from build123d import *

# Parameters (mm, degrees)
SKETCH_2_R          = 5
EXTRUDE_1_DEPTH     = 16
SKETCH_3_R          = 8
EXTRUDE_2_DEPTH     = 7
SKETCH_4_R          = 4
EXTRUDE_3_DEPTH     = 13.25
CUT_EXTRUDE_1_DEPTH = 3
CHAMFER_1_SIZE      = 0.5
SKETCH_6_R          = 4
SKETCH_6_R_2        = 3.5
CUT_EXTRUDE_2_DEPTH = 1


with BuildPart() as part:
    # 草图2 → 凸台-拉伸1 (new body)
    with BuildSketch(Plane.XY):
        Circle(SKETCH_2_R)
    extrude(amount=EXTRUDE_1_DEPTH)

    # 草图3 → 凸台-拉伸2 (add)
    with BuildSketch(Plane.XY.offset(16)):
        Circle(SKETCH_3_R)
    extrude(amount=EXTRUDE_2_DEPTH)

    # 草图4 → 凸台-拉伸3 (add)
    with BuildSketch(Plane(origin=(0, 0, 0), x_dir=(-1, 0, 0), z_dir=(0, 0, -1))):
        Circle(SKETCH_4_R)
    extrude(amount=EXTRUDE_3_DEPTH)

    # 草图5 → 切除-拉伸1 (cut)
    with BuildSketch(Plane.XY.offset(23)):
        Polygon((0, 5.456235198), (-4.72523829, 2.728117599), (-4.72523829, -2.728117599), (0, -5.456235198), (4.72523829, -2.728117599), (4.72523829, 2.728117599), align=None)
    extrude(amount=-CUT_EXTRUDE_1_DEPTH, mode=Mode.SUBTRACT)

    # 倒角1
    chamfer_1_edges = [part.edges().sort_by_distance(p)[0] for p in [
        (4, 0, -13.25),
    ]]
    chamfer(chamfer_1_edges, length=CHAMFER_1_SIZE)

    # 草图6 → 切除-拉伸2 (cut)
    with BuildSketch(Plane(origin=(0, 0, 0), x_dir=(-1, 0, 0), z_dir=(0, 0, -1))):
        Circle(SKETCH_6_R)
        Circle(SKETCH_6_R_2, mode=Mode.SUBTRACT)
    extrude(amount=CUT_EXTRUDE_2_DEPTH, mode=Mode.SUBTRACT)


solid = part.part
Geometry check sheet. Reference: the model listing, model coordinates, mm. A direction names the side the tool comes from. Give positions to 0.01 mm unless a question says otherwise; leave off trailing zeros. Write each loop counter-clockwise with the first axis right and the second up, starting at its lowest first coordinate (ties: lowest second). Pieces come first, ordered by that corner, then holes. Notation, with made-up numbers: (-5.5, 34.25) - (52.5, 34.25) arc R24 ccw to (52.5, 65.25) - close; hole circle Ø1 at (1.5, -21.5). An arc over 180 degrees is marked (long way). Put each result on its own line as item: value.
1. Sectioned sample at D-D, the plane y = 4.5. Enter the section's corners in (x, z).
Ans:
outline: (-6.61, 16) - (-2.18, 16) - (-2.18, 0) - (2.18, 0) - (2.18, 16) - (6.61, 16) - (6.61, 23) - (1.66, 23) - (1.66, 20) - (-1.66, 20) - (-1.66, 23) - (-6.61, 23) - close
2. Sectioned sample at B-B, the plane z = 18. Enter the section's corners in (x, y), plus the area to 3 significant figures.
Ans:
outline: circle Ø16 at (0, 0)
area: 201 mm²
3. Thickness scan on line 1 (Z direction, x = -1.5, y = -4); line 2 (Z direction, x = -2.75, y = 5); line 3 (Y direction, x = -3, z = 21). Record the ranges inside material, lowest first.
Ans:
line 1: z = 0 to 20
line 2: z = 16 to 23
line 3: y = -7.42 to -3.72, 3.72 to 7.42
4. Sectioned sample at A-A, the plane y = 0. Enter the section's corners in (x, z).
Ans:
outline: (-8, 16) - (-5, 16) - (-5, 0) - (-3.5, 0) - (-3.5, -1) - (-4, -1) - (-4, -12.75) - (-3.5, -13.25) - (3.5, -13.25) - (4, -12.75) - (4, -1) - (3.5, -1) - (3.5, 0) - (5, 0) - (5, 16) - (8, 16) - (8, 23) - (4.73, 23) - (4.73, 20) - (-4.73, 20) - (-4.73, 23) - (-8, 23) - close
5. Go/stop test with flat-tipped pins: pin 1 (5 mm diameter, centred on y = -1.5, z = -5, fed in from -X); pin 2 (6 mm diameter, centred on x = 1.5, z = 3, fed in from +Y); pin 3 (7.5 mm diameter, centred on x = 1.5, y = -2.5, fed in from +Z); pin 4 (5 mm diameter, centred on x = -3, z = 17, fed in from +Y). Record where each tip stops, or that it passes through.
Ans:
pin 1: stops at x = -4
pin 2: stops at y = 5
pin 3: stops at z = 23
pin 4: stops at y = 7.98
6. Sectioned sample at C-C, the plane x = 6. Enter the section's corners in (y, z).
Ans:
outline: (-5.29, 16) - (5.29, 16) - (5.29, 23) - (-5.29, 23) - close
7. Draft check along X on faces 5 (the flat face through (0, 0, 20)), 6 (the cylindrical face through (-1.73, -7.81, 19.45)), 7 (the flat face through (0, 0, -13.25)). Enter one of: +X half, -X half, draft (parallel to the pull), parting line (faces both ways), or undercut.
Ans:
face 5: undercut
face 6: parting line
face 7: draft
8. Set-up check for faces 1 (the cylindrical face through (-1.08, -4.88, 7.89)), 2 (the flat face through (2.2, -3.3, 0)), 3 (the flat face through (-4.725, 0, 22)), 4 (the flat face through (3, 4, 23)): record each of +Z, -Z, +X, -X, +Y, -Y from which the full face is reachable in a straight line by a thin tool's end or side.
Ans:
face 1: -Z
face 2: none
face 3: +Z
face 4: +Z, +X, -X, +Y, -Y
